Geometry check sheet. Reference: the model listing, model coordinates, mm. Face numbers are marked on the shaded views. A direction names the side the tool comes from. Round coordinates to 2 decimals unless told otherwise and drop trailing zeros. Write each loop counter-clockwise with the first axis right and the second up, starting at its lowest first coordinate (ties: lowest second). Pieces come first, ordered by that corner, then holes. Notation, with made-up numbers: M 18.25,0.25 L 58.25,0.25 A22 ccw 58.25,27.25 Z; hole C -32.5,4.25 d8. An arc over 180 degrees is marked long. One line per item, written item: value. Start each with the question number.
1. Section check B-B (y = -55). Record the boundary of the cut face in (x, z).
2. Section check C-C (z = 30.25). Record the boundary of the cut face in (x, y), and give its area (3 significant figures).
3. Section check D-D (z = 34.75). Record the boundary of the cut face in (x, y).
4. Access from +Z, -Z, +X, -X, +Y, -Y to the whole of each face (thin tool, end or side, straight path). Record for the marked faces 4 and 5.
5. Depth check by flat-ended pin: P1, Ø1.5, axis at x = 16, y = -55.5, coming from the -Z side; P2, Ø1.5, axis at y = -58.5, z = 34, coming from the -X side. Enter the tip coordinate at first touch or a pass-through.
6. Scan lines: probe 1 along Y at (x, z) = (15.5, 28.9); probe 2 along X at (y, z) = (-55, 28.95); probe 3 along Z at (x, y) = (18.5, -54.25). Record each from-to range of solid material in increasing order. Write a range as [from, to].
7. Section check A-A (z = 27.75). Record the boundary of the cut face in (x, y).
8. Release check for a two-part mould opening along X. For the marked faces 1, 2 and 3 record: pulls with the +X half, pulls with the -X half, needs draft (parallel to the pull), parting line crosses it, or undercut.
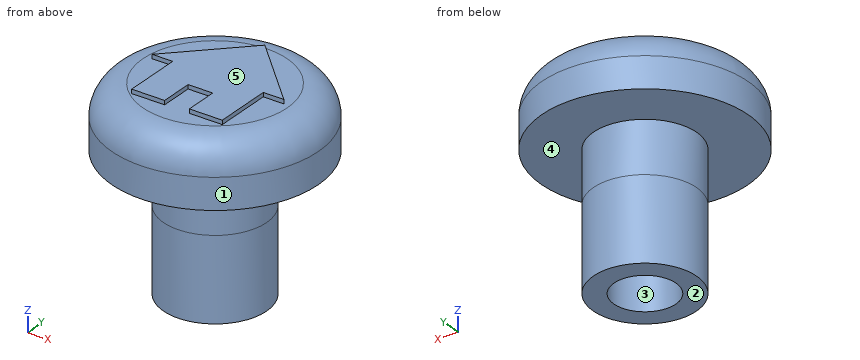
from build123d import *

# Parameters (mm, degrees)
SKETCH046_R     = 2.5
PAD023_DEPTH    = 2.5
SKETCH047_R     = 5
PAD024_DEPTH    = 3
FILLET003_R     = 1.5
SKETCH049_R     = 2.5
PAD025_DEPTH    = 4
SKETCH050_R     = 1.5
POCKET026_DEPTH = 4
PAD051_DEPTH    = 0.2


with BuildPart() as part:
    # Sketch046 → Pad023 (new body)
    with BuildSketch(Plane(origin=(0, 0, 30), x_dir=(1, 0, 0), z_dir=(0, 0, -1))):
        with Locations((101, 55)):
            Circle(SKETCH046_R)
    extrude(amount=-PAD023_DEPTH)

    # Sketch047 (on Face3 of Pad023) → Pad024 (join)
    with BuildSketch(Plane.XY.offset(32.5)):
        with Locations((101, -55)):
            Circle(SKETCH047_R)
    extrude(amount=PAD024_DEPTH)

    # Fillet003
    fillet003_edges = [part.edges().sort_by_distance(p)[0] for p in [
        (96, -55, 35.5),
    ]]
    fillet(fillet003_edges, radius=FILLET003_R)

    # Sketch049 → Pad025 (join)
    with BuildSketch(Plane(origin=(0, 0, 30), x_dir=(1, 0, 0), z_dir=(0, 0, -1))):
        with Locations((101, 55)):
            Circle(SKETCH049_R)
    extrude(amount=PAD025_DEPTH)

    # Sketch050 (on Face17 of Pad025) → Pocket026 (cut)
    with BuildSketch(Plane(origin=(0, 0, 26), x_dir=(1, 0, 0), z_dir=(0, 0, -1))):
        with Locations((101, 55)):
            Circle(SKETCH050_R)
    extrude(amount=-POCKET026_DEPTH, mode=Mode.SUBTRACT)


with BuildPart() as part_1:
    # Body002 placement: moved
    add(part.part.moved(Location((75, 0, 0))))

    # Sketch085 (on Face4 of Clone003) → Pad051 (new body)
    with BuildSketch(Plane(origin=(176, -55, 35.5), x_dir=(1, 0, 0), z_dir=(0, 0, 1))):
        Polygon((-0.6, -2.6), (-0.6, -1), (0.6, -1), (0.6, -2.6), (2.2, -2.6), (2.2, 0.2), (3.2, 0.2), (0, 3.4), (-3.2, 0.2), (-2.2, 0.2), (-2.2, -2.6), align=None)
    extrude(amount=PAD051_DEPTH)


with BuildPart() as part_2:
    # Body009 placement: moved
    add(part_1.part.moved(Location((-160.5, 0, 0))))


solid = part_2.part
Result sheet:
1. outline: M 10.5,32.5 L 13,32.5 L 13,26 L 14,26 L 14,30 L 17,30 L 17,26 L 18,26 L 18,32.5 L 20.5,32.5 L 20.5,34 A1.5 ccw 19,35.5 L 17.7,35.5 L 17.7,35.7 L 13.3,35.7 L 13.3,35.5 L 12,35.5 A1.5 ccw 10.5,34 Z
2. outline: C 15.5,-55 d5
2. area: 19.6 mm2
3. outline: C 15.5,-55 d9.6
4. face 4: -Z
4. face 5: +Z, +X, -X, +Y, -Y
5. P1: stops at z = 30
5. P2: stops at x = 11.32
6. probe 1: y = [-57.5, -56.5], [-53.5, -52.5]
6. probe 2: x = [13, 14], [17, 18]
6. probe 3: z = [32.5, 35.5]
7. outline: C 15.5,-55 d5; hole C 15.5,-55 d3
8. face 1: parting line crosses it
8. face 2: needs draft
8. face 3: undercut
